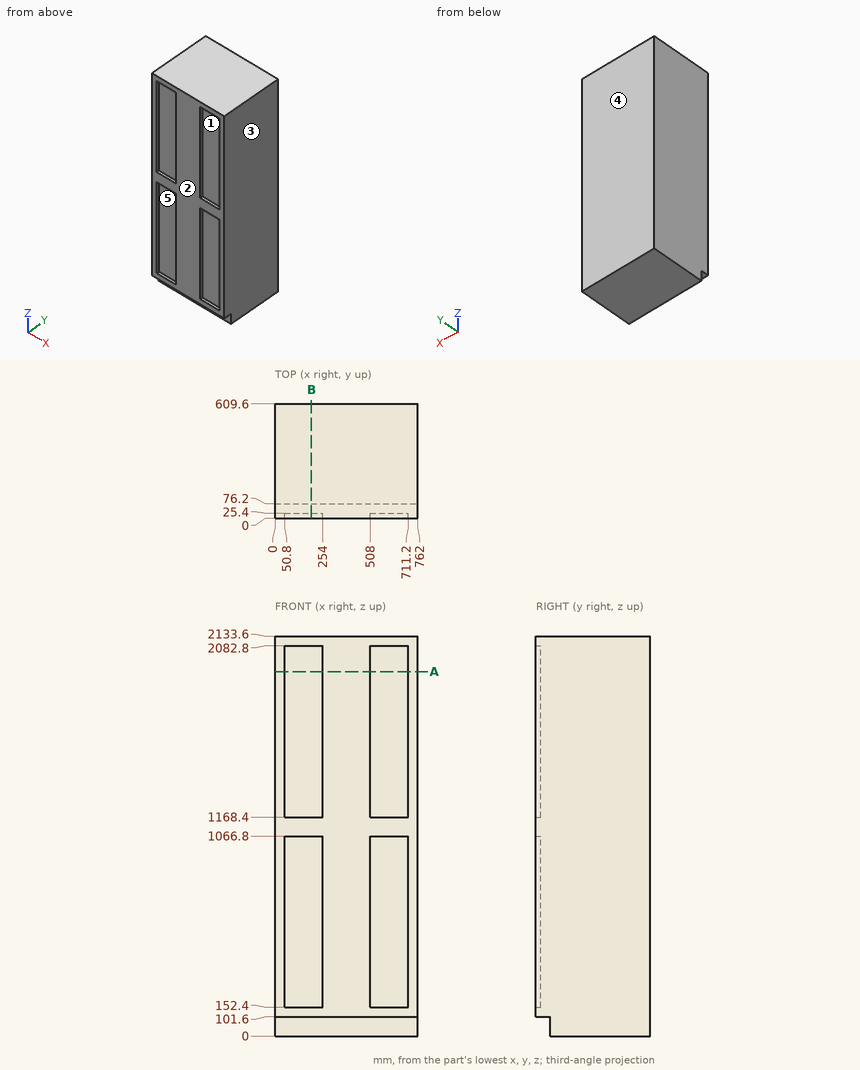
Here's the drawing with two shaded views (mm, measured from the low corner). I have some questions. A direction names the side the tool comes from. Coordinates: 2 decimals unless noted, no trailing zeros. Loops run counter-clockwise (first coordinate to the right, second up) from the corner with the lowest first, then second, coordinate; pieces in that order, holes last. Notation, with made-up numbers: (-40, 85) -> (16, 85) arc R15 ccw to (16, 105) -> close; hole circle Ø11 at (-34.5, 59.5). An arc over 180 degrees is marked (long way). Answer in a Markdown table with one row per item.
(1) If I drill on probe 1 along Y at (x, z) = (696, 1353); probe 2 along Y at (x, z) = (474, 85.5); probe 3 along Z at (x, y) = (185.5, 60.5), over which ranges is the centre line in solid material (lowest first)?
Results found:
| item | result |
|---|---|
| probe 1 | y = 25.4 to 609.6 |
| probe 2 | y = 76.2 to 609.6 |
| probe 3 | z = 101.6 to 2133.6 |
(2) For the marked faces 4 and 5, which set-ups out of +Z, -Z, +X, -X, +Y, -Y let a thin tool reach every point of the face, with its end or its side?
Results found:
| item | result |
|---|---|
| face 4 | +Z, -Z, +X, -X, +Y |
| face 5 | -Y |
(3) Will this pin go through, and if not, where does the flat tip stop? pin 1 Ø12.5 at (x, y) = (183, 15.5) entering from -Z.
Results found:
| item | result |
|---|---|
| pin 1 | stops at z = 101.6 |
(4) Imagine slicing it at B-B (x = 193.5). List the corners of the cut face in (y, z) for me.
Results found:
| item | result |
|---|---|
| outline | (0, 101.6) -> (76.2, 101.6) -> (76.2, 0) -> (609.6, 0) -> (609.6, 2133.6) -> (0, 2133.6) -> (0, 2082.8) -> (25.4, 2082.8) -> (25.4, 1168.4) -> (0, 1168.4) -> (0, 1066.8) -> (25.4, 1066.8) -> (25.4, 152.4) -> (0, 152.4) -> close |
(5) Imagine slicing it at A-A (z = 1944). List the corners of the cut face in (x, y) for me.
Results found:
| item | result |
|---|---|
| outline | (0, 0) -> (50.8, 0) -> (50.8, 25.4) -> (254, 25.4) -> (254, 0) -> (508, 0) -> (508, 25.4) -> (711.2, 25.4) -> (711.2, 0) -> (762, 0) -> (762, 609.6) -> (0, 609.6) -> close |
(6) Thinking about a two-plate mould opening in X: for the marked faces 1, 2 and 3, which applies, released by +X, released by -X, zero draft, split by the parting line, or undercut?
Results found:
| item | result |
|---|---|
| face 1 | undercut |
| face 2 | zero draft |
| face 3 | released by +X |
